from build123d import *

# Parameters (mm, degrees)
SKETCH_1_W      = 30
SKETCH_1_H      = 20
EXTRUDE_1_DEPTH = 40
SKETCH_2_R      = 2
EXTRUDE_2_DEPTH = 5
SKETCH_3_RX     = 29.20442212
SKETCH_3_RY     = 5
EXTRUDE_4_DEPTH = 10
EXTRUDE_5_DEPTH = 2


with BuildPart() as part:
    # 草图1 → 凸台-拉伸1 (new body)
    with BuildSketch(Plane.XY):
        with Locations((15, 10)):
            Rectangle(SKETCH_1_W, SKETCH_1_H)
    extrude(amount=EXTRUDE_1_DEPTH)

    # 草图2 → 凸台-拉伸2 (add)
    with BuildSketch(Plane.ZY):
        with Locations(Location((30, 10, 0), (0, 0, 180))):
            Circle(SKETCH_2_R)
    extrude(amount=EXTRUDE_2_DEPTH)

    # 草图3 → 凸台-拉伸4 (add)
    with BuildSketch(Plane.ZY.offset(5)):
        with Locations(Location((30, 10), (0, 0, -58.183129666))):
            Ellipse(SKETCH_3_RX, SKETCH_3_RY)
    extrude(amount=EXTRUDE_4_DEPTH)

    # 草图4 → 凸台-拉伸5 (add)
    with BuildSketch(Plane.ZY.offset(15)):
        with BuildLine():
            add(Edge.make_bspline(
                [(44.671665843, -16.341862431), (45.731147297, -16.721716463), (46.343386543, -16.341862431)],
                knots=[6.044161849, 6.044161849, 6.044161849, 6.283185307, 6.283185307, 6.283185307], degree=2, weights=[1, 0.99286697, 1]))
            Line((46.343386543, -16.341862431), (44.671665843, -16.341862431))
        make_face()
        with BuildLine():
            Line((44.671665843, -16.341862431), (46.343386543, -16.341862431))
            add(Edge.make_bspline(
                [(46.343386543, -16.341862431), (47.091960208, -15.877421892), (47.119167153, -14.320823946)],
                knots=[0, 0, 0, 0.29156576, 0.29156576, 0.29156576], degree=2, weights=[1, 0.989392482, 1]))
            add(Edge.make_bspline(
                [(47.119167153, -14.320823946), (47.153377166, -12.363557646), (46.056833567, -8.932081728)],
                knots=[0.29156576, 0.29156576, 0.29156576, 0.656688827, 0.656688827, 0.656688827], degree=2, weights=[1, 0.983381875, 1]))
            Line((46.056833567, -8.932081728), (45.971258289, -13.31870573))
            add(Edge.make_bspline(
                [(45.396747079, -14.816092575), (45.948727857, -14.473624944), (45.971258289, -13.31870573)],
                knots=[3.141592654, 3.141592654, 3.141592654, 3.399981292, 3.399981292, 3.399981292], degree=2, weights=[1, 0.991666016, 1]))
            add(Edge.make_bspline(
                [(44.16063068, -14.816092575), (44.945440411, -15.096098568), (45.396747079, -14.816092575)],
                knots=[2.929941094, 2.929941094, 2.929941094, 3.141592654, 3.141592654, 3.141592654], degree=2, weights=[1, 0.994405676, 1]))
            Line((44.16063068, -14.816092575), (42.129626505, -14.816092575))
            add(Edge.make_bspline(
                [(42.129626505, -14.816092575), (43.598799221, -15.957209438), (44.671665843, -16.341862431)],
                knots=[5.802147853, 5.802147853, 5.802147853, 6.044161849, 6.044161849, 6.044161849], degree=2, weights=[1, 0.992687583, 1]))
        make_face()
        with BuildLine():
            Line((0, -16.341862431), (44.671665843, -16.341862431))
            add(Edge.make_bspline(
                [(42.129626505, -14.816092575), (43.598799221, -15.957209438), (44.671665843, -16.341862431)],
                knots=[5.802147853, 5.802147853, 5.802147853, 6.044161849, 6.044161849, 6.044161849], degree=2, weights=[1, 0.992687583, 1]))
            Line((42.129626505, -14.816092575), (0, -14.816092575))
            Line((0, -14.816092575), (0, -16.341862431))
        make_face()
        with BuildLine():
            add(Edge.make_bspline(
                [(47.119167153, -14.320823946), (47.153377166, -12.363557646), (46.056833567, -8.932081728)],
                knots=[0.29156576, 0.29156576, 0.29156576, 0.656688827, 0.656688827, 0.656688827], degree=2, weights=[1, 0.983381875, 1]))
            Line((47.119167153, -14.320823946), (48.165155486, 45.523575701))
            Line((48.165155486, 45.523575701), (47.119167153, 45.523575701))
            Line((47.119167153, 45.523575701), (46.056833567, -8.932081728))
        make_face()
    extrude(amount=-EXTRUDE_5_DEPTH)


solid = part.part
Source: CAD feature listing. Evaluate the final solid. Frame: model axes, mm. A direction names the side the tool comes from. Coordinates: 2 decimals unless noted, no trailing zeros. Order: outer loops, then holes, each group sorted by start corner. A loop starts at its lowest first (then second) coordinate and runs counter-clockwise, first axis right, second up.
Item 1: Material intervals for line 1 (X direction, y = 13, z = 27.5); line 2 (Z direction, x = 2, y = 15); line 3 (Y direction, x = 17, z = 32), sorted ascending.
Output values:
line 1: x = -15 to -5, 0 to 30
line 2: z = 0 to 40
line 3: y = 0 to 20
Item 2: Cut plane A-A (z = 12). Return loops of the section in (x, y), plus the area to 3 significant figures.
Output values:
outline: (-15, -16.34) - (-13, -16.34) - (-13, -14.82) - (-15, -14.82) - close; (0, 0) - (30, 0) - (30, 20) - (0, 20) - close
area: 603 mm2
Item 3: Set-up query: faces 1 (the face through (15, 0, 20)), 2 (the face through (-2.465, 9.399, 28.092)), 3 (the face through (15, 20, 20)), 4 (the face through (-14, -16.342, 22)). Return all of +Z, -Z, +X, -X, +Y, -Y with unobstructed straight access to the full face (end or side cutting, diameter ignored); none if empty.
Output values:
face 1: +Z, -Z, +X, -Y
face 2: none
face 3: +Z, -Z, +X, +Y
face 4: -Z, +X, -X, -Y
Item 4: Cut plane B-B (z = 37.5). Count the separate pieces of the cut face and the enclosed holes in it, plus the area to 3 significant figures.
Output values:
separate pieces: 3
enclosed holes: 0
area: 764 mm2
Item 5: Pull-direction query (X, two-part tool) for faces 5 (the face through (15, 10, 40)), 6 (the face through (-5, 9, 28)), 7 (the face through (-15, 8, 31)), 8 (the face through (30, 10, 20)); classes: pulls with the +X half, pulls with the -X half, needs draft (parallel to the pull), parting line crosses it, or undercut.
Output values:
face 5: needs draft
face 6: undercut
face 7: pulls with the -X half
face 8: pulls with the +X half
Item 6: First-contact query: P1, Ø6, axis at x = 18, y = 7.5, coming from the +Z side; P2, Ø8, axis at x = 23, z = 12, coming from the +Y side; P3, Ø1.6, axis at x = -13.5, z = 24, coming from the -Y side; P4, Ø10, axis at x = 7, y = 14, coming from the -Z side. Flat tips, straight axial feed; report the tip coordinate or a pass-through.
Output values:
P1: stops at z = 40
P2: stops at y = 20
P3: stops at y = -16.34
P4: stops at z = 0
Item 7: Cut plane C-C (x = 12.5). Return loops of the section in (y, z).
Output values:
outline: (0, 0) - (20, 0) - (20, 40) - (0, 40) - close
